Build history of the part. All positions in model axes, mm. Coordinates: 2 decimals unless noted, no trailing zeros. Loops run counter-clockwise (first coordinate to the right, second up) from the corner with the lowest first, then second, coordinate; pieces in that order, holes last.
(1) Slice it at C-C (z = 2.5). Give the cut face in (x, y), and give its area (3 significant figures).
(2) Slice it at D-D (y = 70). Give the cut face in (x, z).
(3) Two-plate mould, pull along Y, no slides. Class faces 1 (the face through (11.15, 165.58, 5.07)), 2 (the face through (48, 177.8, 5)), 3 (the face through (2.846, 90.145, 5.07)): pulls with the +Y half, pulls with the -Y half, needs draft (parallel to the pull), parting line crosses it, or undercut.
(4) Slice it at B-B (y = 10). Give the cut face in (x, z), and give its area (3 significant figures).
(5) Flat gauge pins, fed straight in: P1, Ø11, axis at x = 57.15, y = 19.05, coming from the +Z side; P2, Ø6, axis at y = 33, z = 2.5, coming from the -X side. Where does each tip first touch, or does it go through?
(6) Wall check: L1, parallel to Y at x = 85.25, z = 7.75; L2, parallel to Y at x = 9.5, z = 5.75; L3, parallel to X at y = 167.8, z = 7.5. Give the ranges that are in metal, low to high.
(7) Slice it at A-A (x = 85.25). Give the cut face in (y, z), and give its area (3 significant figures).
Autodesk Inventor part; units mm, degrees
ref_plane "YZ Plane" through (0, 0, 0) normal (1, 0, 0) x (0, 1, 0)
ref_plane "XZ Plane" through (0, 0, 0) normal (0, 1, 0) x (-1, 0, 0)
ref_plane "XY Plane" through (0, 0, 0) normal (0, 0, 1) x (1, 0, 0)
sketch "Sketch1" plane through (0, 0, 0) normal (0, 0, 1) x (1, 0, 0)
  line L0 (0, 0) -> (95.25, 0)
  line L1 (95.25, 0) -> (95.25, 177.8)
  line L2 (95.25, 177.8) -> (0, 177.8)
  line L3 (0, 177.8) -> (0, 0)
  dimension "d0" = 95.25
  dimension "d1" = 177.8
extrude "Extrusion1" add sketch "Sketch1" along normal blind 10
sketch "Sketch2" plane through (0, 177.8, 0) normal (0, 1, 0) x (1, 0, 0)
  line L0 (0, -10) -> (95.25, -10)
  line L1 (0, -10) -> (5.7735, 0)
  line L2 (0, 0) -> (95.25, 0)
  line L3 (0, 0) -> (0, -10)
  line L4 (5.7735, 0) -> (0, 0)
  dimension "d4" = 30
extrude "Extrusion2" cut sketch "Sketch2" against normal through all
sketch "Sketch3" plane through (0, 0, 10) normal (0, 0, 1) x (1, 0, 0)
  line L0 (0, 0) -> (95.25, 0) construction
  line L1 (95.25, 0) -> (95.25, 177.8) construction
  line L2 (95.25, 177.8) -> (0, 177.8) construction
  line L3 (0, 177.8) -> (0, 0) construction
  line L4 (10, 10) -> (85.25, 10) construction
  line L5 (85.25, 10) -> (85.25, 167.8) construction
  line L6 (85.25, 167.8) -> (10, 167.8) construction
  line L7 (10, 167.8) -> (10, 10) construction
  circle A0 centre (10, 167.8) radius 2.5
  circle A1 centre (85.25, 167.8) radius 2.5
  circle A2 centre (85.25, 10) radius 2.5
  circle A3 centre (10, 10) radius 2.5
  dimension "d7" = 10
  dimension "d8" = 5
  dimension "d9" = 5
  dimension "d10" = 5
  dimension "d11" = 5
extrude "Extrusion3" cut sketch "Sketch3" against normal through all
sketch "Sketch4" plane through (0, 0, 10) normal (0, 0, 1) x (1, 0, 0)
  circle A0 centre (57.15, 19.05) radius 6
  line L0 (95.25, 177.8) -> (0, 177.8)
  line L1 (95.25, 0) -> (95.25, 177.8)
  line L2 (0, 0) -> (95.25, 0)
  dimension "d14" = 12
  dimension "d16" = 38.1
  dimension "d19" = 19.05
extrude "Extrusion4" cut sketch "Sketch4" against normal through all
properties part number "BA09" material "ABS Plastic"
Response values:
1. outline: (4.33, 0) - (95.25, 0) - (95.25, 177.8) - (4.33, 177.8) - close; hole circle Ø5 at (10, 10); hole circle Ø5 at (10, 167.8); hole circle Ø12 at (57.15, 19.05); hole circle Ø5 at (85.25, 10); hole circle Ø5 at (85.25, 167.8)
1. area: 16,000 mm2
2. outline: (0, 10) - (5.77, 0) - (95.25, 0) - (95.25, 10) - close
3. face 1: undercut
3. face 2: pulls with the +Y half
3. face 3: needs draft
4. outline: (0, 10) - (5.77, 0) - (7.5, 0) - (7.5, 10) - close; (12.5, 0) - (82.75, 0) - (82.75, 10) - (12.5, 10) - close; (87.75, 0) - (95.25, 0) - (95.25, 10) - (87.75, 10) - close
4. area: 824 mm2
5. P1: passes through
5. P2: stops at x = 2.6
6. L1: y = 0 to 7.5, 12.5 to 165.3, 170.3 to 177.8
6. L2: y = 0 to 7.55, 12.45 to 165.35, 170.25 to 177.8
6. L3: x = 1.44 to 7.5, 12.5 to 82.75, 87.75 to 95.25
7. outline: (0, 0) - (7.5, 0) - (7.5, 10) - (0, 10) - close; (12.5, 0) - (165.3, 0) - (165.3, 10) - (12.5, 10) - close; (170.3, 0) - (177.8, 0) - (177.8, 10) - (170.3, 10) - close
7. area: 1,680 mm2
